Work out the finished part from the listing and answer in its coordinate system (mm). Face numbers are marked on the shaded views. A direction names the side the tool comes from. Round coordinates to 2 decimals unless told otherwise and drop trailing zeros. Order: outer loops, then holes, each group sorted by start corner. A loop starts at its lowest first (then second) coordinate and runs counter-clockwise, first axis right, second up.
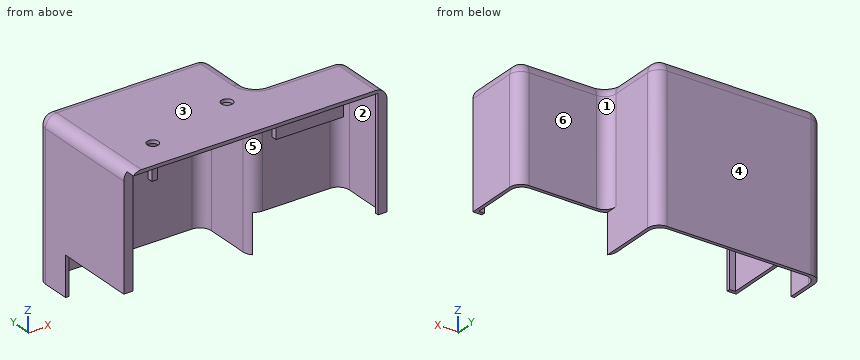
from build123d import *

# Parameters (mm, degrees)
BOSS_EXTRUDE1_DEPTH = 100
BOSS_EXTRUDE2_DEPTH = 3
SKETCH3_R           = 5
CUT_EXTRUDE1_DEPTH  = 3
SKETCH4_W           = 5
SKETCH4_H           = 5
SKETCH4_W_2         = 60
BOSS_EXTRUDE3_DEPTH = 15
BOSS_EXTRUDE4_DEPTH = 35
FILLET2_R           = 10


with BuildPart() as part:
    # Sketch1 → Boss-Extrude1 (new body)
    with BuildSketch(Plane.XY):
        Polygon((-212, 8), (-220, 8), (-220, 116), (-72, 116), (-72, 56), (8, 56), (8, 0), (0, 0), (0, 3), (5, 3), (5, 53), (-75, 53), (-75, 113), (-217, 113), (-217, 11), (-212, 11), align=None)
    extrude(amount=BOSS_EXTRUDE1_DEPTH)

    # Sketch2 → Boss-Extrude2 (add)
    with BuildSketch(Plane.XY.offset(100)):
        Polygon((0, 0), (8, 0), (8, 56), (-72, 56), (-72, 116), (-220, 116), (-220, 8), (-220, 0), align=None)
    extrude(amount=BOSS_EXTRUDE2_DEPTH)

    # Sketch3 → Cut-Extrude1 (cut)
    with BuildSketch(Plane.XY.offset(103)):
        with Locations((-180, 28)):
            Circle(SKETCH3_R)
        with Locations((-100, 48)):
            Circle(SKETCH3_R)
    extrude(amount=-CUT_EXTRUDE1_DEPTH, mode=Mode.SUBTRACT)

    # Sketch4 → Boss-Extrude3 (add)
    with BuildSketch(Plane(origin=(0, 0, 100), x_dir=(-1, 0, 0), z_dir=(0, 0, -1))):
        with Locations((192.5, 10.5)):
            Rectangle(SKETCH4_W, SKETCH4_H)
        with Locations((54.8, 10.5)):
            Rectangle(SKETCH4_W_2, SKETCH4_H)
    extrude(amount=BOSS_EXTRUDE3_DEPTH)

    # Sketch5 → Boss-Extrude4 (add)
    with BuildSketch(Plane(origin=(0, 0, 0), x_dir=(-1, 0, 0), z_dir=(0, 0, -1))):
        Polygon((72, 116), (220, 116), (220, 81), (217, 81), (217, 113), (75, 113), (75, 53), (72, 53), (72, 56), align=None)
    extrude(amount=BOSS_EXTRUDE4_DEPTH)

    # Fillet2
    fillet2_edges = [part.edges().sort_by_distance(p)[0] for p in [
        (-32, 56, 103),
        (-220, 58, 103),
        (8, 28, 103),
        (-72, 86, 103),
        (-146, 116, 103),
        (-220, 116, 34),
        (-217, 113, 32.5),
        (5, 53, 50),
        (8, 56, 51.5),
        (-75, 53, 32.5),
        (-75, 113, 32.5),
        (-72, 56, 51.5),
        (-72, 116, 34),
    ]]
    fillet(fillet2_edges, radius=FILLET2_R)


solid = part.part
Item 1: Find section A-A (x = -180). Write down the section's boundary in (y, z).
Item 2: Find section D-D (y = 78). Write down the section's boundary in (x, z).
Item 3: For a pull along X with two mould halves and no side action, classify the marked faces 1, 2 and 3 as released by +X, released by -X, zero draft, split by the parting line, or undercut.
Item 4: Find section C-C (z = -13). Write down the section's boundary in (x, y), plus the area to 3 significant figures.
Item 5: A tool of negligible diameter and unlimited length cuts with its end or side. For the marked faces 4, 5 and 6, from which of +Z, -Z, +X, -X, +Y, -Y can it reach the whole face along a straight path? Write none if from no direction.
Item 6: Find the intervals of material crossed by line 1 along X through (y, z) = (100, 73); line 2 along X through (y, z) = (73.5, 94); line 3 along Y through (x, z) = (-111, -4.5), in increasing order.
Item 7: Given pin 1 (2.5 mm diameter, centred on x = -217, y = 56, fed in from -Z); pin 2 (7.5 mm diameter, centred on x = -59.5, z = 92.5, fed in from -Y); pin 3 (1.5 mm diameter, centred on x = 2.5, z = 64, fed in from +Y), each flat-ended and moving along its own axis, determine where each tip first touches the part or whether it passes through.
Item 8: Find section B-B (y = 28). Write down the section's boundary in (x, z).
Model answer:
1. outline: (0, 100) - (23, 100) - (23, 103) - (0, 103) - close; (33, 100) - (113, 100) - (113, -35) - (116, -35) - (116, 93) arc R10 ccw to (106, 103) - (33, 103) - close
2. outline: (-220, 0) - (-217, 0) - (-217, 100) - (-75, 100) - (-75, -35) - (-72, -35) - (-72, 93) arc R10 ccw to (-82, 103) - (-210, 103) arc R10 ccw to (-220, 93) - close
3. face 1: released by +X
3. face 2: undercut
3. face 3: zero draft
4. outline: (-220, 81) - (-217, 81) - (-217, 103) arc R10 cw to (-207, 113) - (-85, 113) arc R10 cw to (-75, 103) - (-75, 63) arc R10 ccw to (-72, 55.86) - (-72, 106) arc R10 ccw to (-82, 116) - (-210, 116) arc R10 ccw to (-220, 106) - close
4. area: 705 mm2
5. face 4: +Z, -Z, +X, -X, +Y
5. face 5: -Z
5. face 6: +Z, -Z, +X, +Y
6. line 1: x = -220 to -217, -75 to -72
6. line 2: x = -219.95 to -217, -75 to -72.05
6. line 3: y = 113 to 116
7. pin 1: stops at z = 0
7. pin 2: stops at y = 8
7. pin 3: stops at y = 55.27
8. outline: (-220, 0) - (-217, 0) - (-217, 100) - (-185, 100) - (-185, 103) - (-210, 103) arc R10 ccw to (-220, 93) - close; (-175, 100) - (5, 100) - (5, 0) - (8, 0) - (8, 93) arc R10 ccw to (-2, 103) - (-175, 103) - close
